```python
from build123d import *

# Parameters (mm, degrees)
SKIZZE1_W                       = 680
SKIZZE1_H                       = 280
AUFSATZ_LINEAR_AUSTRAGEN1_DEPTH = 5
SKIZZE2_W                       = 5
SKIZZE2_H                       = 80
AUFSATZ_LINEAR_AUSTRAGEN2_DEPTH = 5
SKIZZE3_W                       = 100
SKIZZE3_H                       = 5
SCHNITT_LINEAR_AUSTRAGEN1_DEPTH = 373.357355238


with BuildPart() as part:
    # Skizze1 → Aufsatz-Linear austragen1 (new body)
    with BuildSketch(Plane(origin=(0, 0, 0), x_dir=(0, 0, -1), z_dir=(1, 0, 0))):
        Rectangle(SKIZZE1_W, SKIZZE1_H)
    extrude(amount=AUFSATZ_LINEAR_AUSTRAGEN1_DEPTH)

    # Skizze2 → Aufsatz-Linear austragen2 (add)
    with BuildSketch(Plane(origin=(5, 0, 0), x_dir=(0, 0, -1), z_dir=(1, 0, 0))):
        with Locations((-342.5, 100)):
            Rectangle(SKIZZE2_W, SKIZZE2_H)
        with Locations((-342.5, -100)):
            Rectangle(SKIZZE2_W, SKIZZE2_H)
        with Locations((342.5, -100)):
            Rectangle(SKIZZE2_W, SKIZZE2_H)
        with Locations((342.5, 100)):
            Rectangle(SKIZZE2_W, SKIZZE2_H)
    extrude(amount=-AUFSATZ_LINEAR_AUSTRAGEN2_DEPTH)

    # Skizze3 → Schnitt-Linear austragen1 (cut, through all)
    with BuildSketch(Plane(origin=(5, 0, 0), x_dir=(0, 0, -1), z_dir=(1, 0, 0))):
        with Locations((200, 137.5)):
            Rectangle(SKIZZE3_W, SKIZZE3_H)
        with Locations((-200, 137.5)):
            Rectangle(SKIZZE3_W, SKIZZE3_H)
        with Locations((0, 137.5)):
            Rectangle(SKIZZE3_W, SKIZZE3_H)
    extrude(amount=-SCHNITT_LINEAR_AUSTRAGEN1_DEPTH, mode=Mode.SUBTRACT)


solid = part.part
```
Read the model definition and answer for the solid it produces. Units are mm, in the model's axes. Coordinates: 2 decimals unless noted, no trailing zeros. Loops run counter-clockwise (first coordinate to the right, second up) from the corner with the lowest first, then second, coordinate; pieces in that order, holes last.
(1) Flat-ended cylindrical pins translate along their axes: pin 1 Ø2.5 at (x, y) = (2.5, -6) entering from -Z; pin 2 Ø3 at (x, z) = (4, 165.5) entering from +Y; pin 3 Ø2.5 at (x, y) = (2.5, 8) entering from +Z. Find the tip coordinate at first contact, or state that the pin passes through.
Solution:
pin 1: stops at z = -340
pin 2: stops at y = 135
pin 3: stops at z = 340
(2) The part is cut by section A-A (z = 194.5). Determine the outline of the cut face in (x, y), and give its area (4 significant figures).
Solution:
outline: (0, -140) - (5, -140) - (5, 135) - (0, 135) - close
area: 1,375 mm2
(3) Consider line 1 along Y through (x, z) = (1.2, -9.5); line 2 along Z through (x, y) = (0.35, -23.5). Determine where each line is inside the solid, lowest interval first.
Solution:
line 1: y = -140 to 135
line 2: z = -340 to 340
